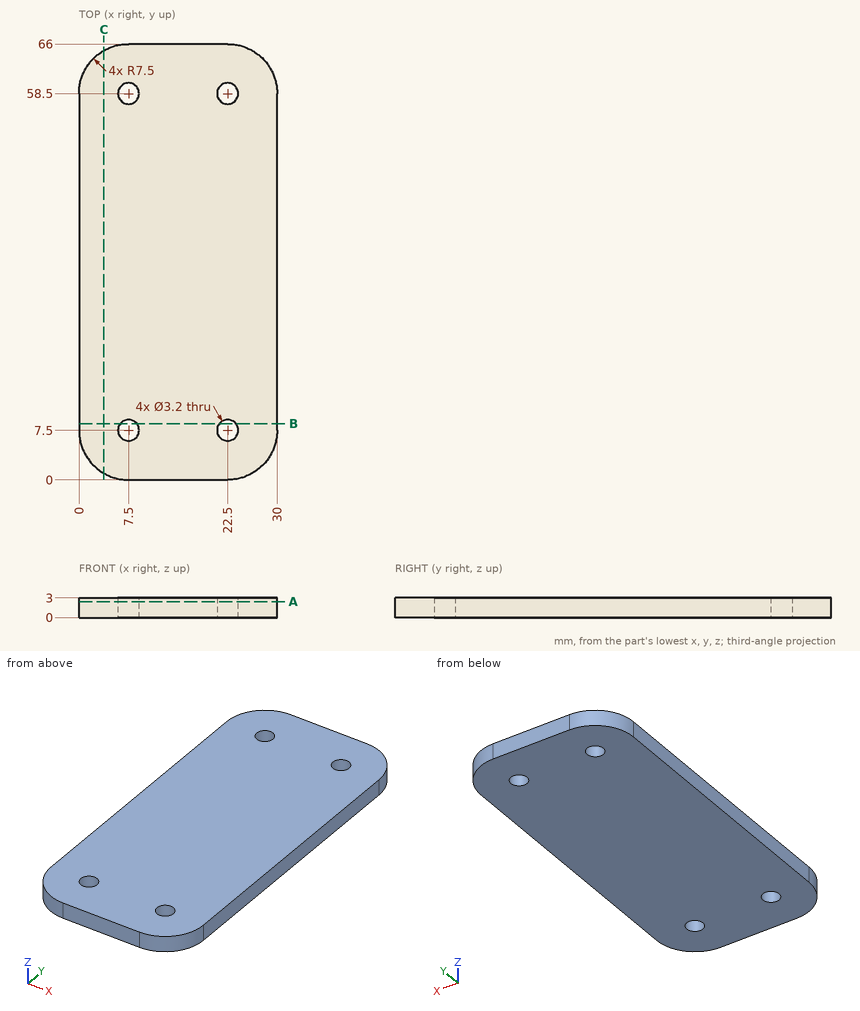
Can you work these out from the drawing? Everything is in mm from the part's minimum corner. Coordinates: 2 decimals unless noted, no trailing zeros. Loops run counter-clockwise (first coordinate to the right, second up) from the corner with the lowest first, then second, coordinate; pieces in that order, holes last. Notation, with made-up numbers: (77, -21) -> (85, -21) arc R20 ccw to (85, -11) -> close; hole circle Ø1 at (51, 9). An arc over 180 degrees is marked (long way). Return JSON: item names as keys, results as strings.
1) If we section it at A-A, the plane z = 2.45: Write out the boundary of the cut face in (x, y), then the cut area to 3 significant figures.
Results below:
{"outline": "(0, 7.5) arc R7.5 ccw to (7.5, 0) -> (22.5, 0) arc R7.5 ccw to (30, 7.5) -> (30, 58.5) arc R7.5 ccw to (22.5, 66) -> (7.5, 66) arc R7.5 ccw to (0, 58.5) -> close; hole circle Ø3.2 at (7.5, 7.5); hole circle Ø3.2 at (7.5, 58.5); hole circle Ø3.2 at (22.5, 7.5); hole circle Ø3.2 at (22.5, 58.5)", "area": "1,900 mm²"}
2) I need wall thicknesses on line 1 (Y direction, x = 22.5, z = 1.8); line 2 (Y direction, x = 8.75, z = 1.3); line 3 (Y direction, x = 2.25, z = 1.95). Which ranges of each line are inside material? Lowest first, please. Write a range as from..to.
Results below:
{"line 1": "0..5.9, 9.1..56.9, 60.1..66", "line 2": "0..6.5, 8.5..57.5, 59.5..66", "line 3": "2.14..63.86"}
3) If we section it at B-B, the plane y = 8.5: Write out the boundary of the cut face in (x, z).
Results below:
{"outline": "(0, 0) -> (6.25, 0) -> (6.25, 3) -> (0, 3) -> close; (8.75, 0) -> (21.25, 0) -> (21.25, 3) -> (8.75, 3) -> close; (23.75, 0) -> (30, 0) -> (30, 3) -> (23.75, 3) -> close"}
4) If we section it at C-C, the plane x = 3.75: Write out the boundary of the cut face in (y, z).
Results below:
{"outline": "(1, 0) -> (65, 0) -> (65, 3) -> (1, 3) -> close"}
